Check sheet for the drawn part. Datum: minimum x, y, z corner. Units: mm. Give positions to 0.01 mm unless a question says otherwise; leave off trailing zeros. Order: outer loops, then holes, each group sorted by start corner. A loop starts at its lowest first (then second) coordinate and runs counter-clockwise, first axis right, second up. Notation, with made-up numbers: M 84,57.5 L 114,57.5 A17 cw 114,79.5 Z; hole C 50.5,-25.75 d1. An arc over 180 degrees is marked long. Put each result on its own line as item: value. Start each with the question number.
Q1. Section check A-A on y = 20. Record the cut outline in (x, z).
Q2. Section check D-D on x = 28.5. Record the cut outline in (y, z), then the cut area to 3 significant figures.
Q3. Section check C-C on z = 1.75. Record the cut outline in (x, y).
Q4. Section check B-B on x = 130. Record the cut outline in (y, z), then the cut area to 3 significant figures.
Q5. Material ranges on L1, parallel to Y at x = 30, z = 4.75; L2, parallel to X at y = 24, z = 2.5; L3, parallel to X at y = 16.5, z = 0.75, recorded low to high.
Q6. Go/stop test with a flat-tipped pin: pin 1 (6 mm diameter, centred on x = 130, y = 20, fed in from +Z). Record where the tip stops, or that it passes through.
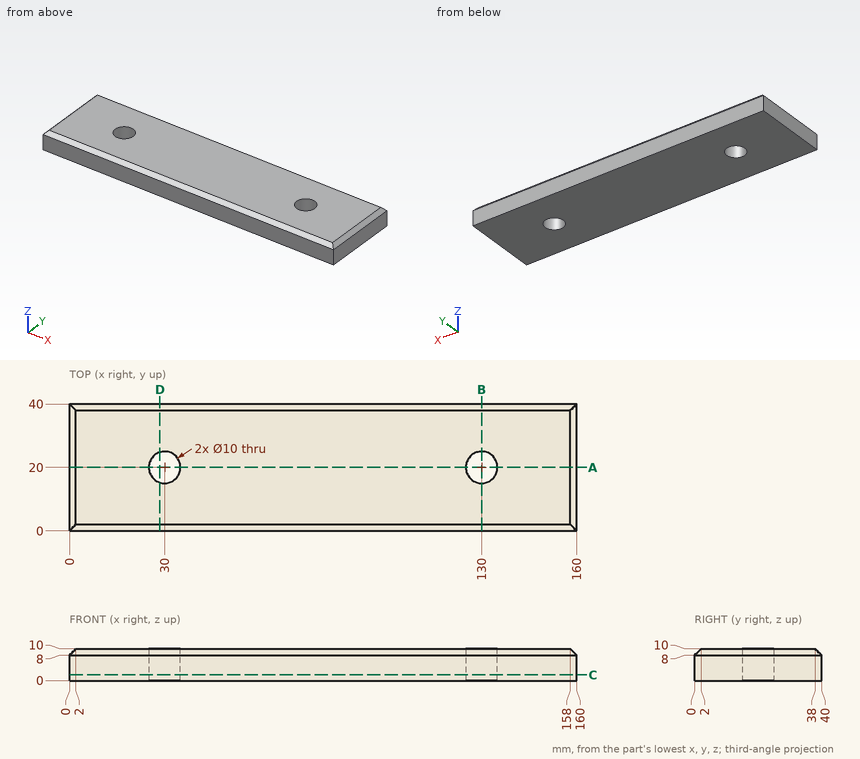
Results found:
1. outline: M 0,0 L 25,0 L 25,10 L 2,10 L 0,8 Z; M 35,0 L 125,0 L 125,10 L 35,10 Z; M 135,0 L 160,0 L 160,8 L 158,10 L 135,10 Z
2. outline: M 0,0 L 15.23,0 L 15.23,10 L 2,10 L 0,8 Z; M 24.77,0 L 40,0 L 40,8 L 38,10 L 24.77,10 Z
2. area: 301 mm^2
3. outline: M 0,0 L 160,0 L 160,40 L 0,40 Z; hole C 30,20 d10; hole C 130,20 d10
4. outline: M 0,0 L 15,0 L 15,10 L 2,10 L 0,8 Z; M 25,0 L 40,0 L 40,8 L 38,10 L 25,10 Z
4. area: 296 mm^2
5. L1: y = 0 to 15, 25 to 40
5. L2: x = 0 to 27, 33 to 127, 133 to 160
5. L3: x = 0 to 26.43, 33.57 to 126.43, 133.57 to 160
6. pin 1: passes through
